```python
from build123d import *

# Parameters (mm, degrees)
SKETCH001_W  = 100
SKETCH001_H  = 80
PAD_DEPTH    = 50
SKETCH_R     = 10
POCKET_DEPTH = 20
SKETCH002_W  = 25
SKETCH002_H  = 50
PAD001_DEPTH = 10


with BuildPart() as part:
    # Sketch001 → Pad (new body)
    with BuildSketch(Plane.XZ):
        Rectangle(SKETCH001_W, SKETCH001_H)
    extrude(amount=-PAD_DEPTH)

    # Sketch → Pocket (cut)
    with BuildSketch(Plane.XZ):
        with Locations((-20, 15)):
            Circle(SKETCH_R)
    extrude(amount=-POCKET_DEPTH, mode=Mode.SUBTRACT)

    # Sketch002 → Pad001 (join)
    with BuildSketch(Plane.XZ):
        with Locations((27.5, -40)):
            Rectangle(SKETCH002_W, SKETCH002_H)
    extrude(amount=-PAD001_DEPTH)


solid = part.part
```
Source: CAD feature listing. Evaluate the final solid. Frame: model axes, mm. A direction names the side the tool comes from. Give positions to 0.01 mm unless a question says otherwise; leave off trailing zeros. Order: outer loops, then holes, each group sorted by start corner. A loop starts at its lowest first (then second) coordinate and runs counter-clockwise, first axis right, second up.
(1) Pull-direction query (X, two-part tool) for faces 1 (the face through (-1, 0, 0)), 2 (the face through (-20, 20, 15)), 3 (the face through (40, 5, -53)); classes: +X half, -X half, draft (parallel to the pull), parting line (faces both ways), or undercut.
(2) Section query A-A (z = 15). Return the cut outline in (x, y), plus the area to 3 significant figures.
(3) Section query C-C (x = -20). Return the cut outline in (y, z), plus the area to 3 significant figures.
(4) Section query B-B (y = 7). Return the cut outline in (x, z).
(5) Material intervals for line 1 along Z through (x, y) = (-20, 13.25); line 2 along Z through (x, y) = (20.5, 43), sorted ascending.
(6) Access query for faces 4 (the face through (-10.46, 9.86, 18)), 5 (the face through (27, 10, -52)), 6 (the face through (-50, 25, -1)), 7 (the face through (15, 5, -53)). Directions: +Z, -Z, +X, -X, +Y, -Y. A direction counts if a zero-diameter tool reaches every point of the face in a straight line with its end or side. Return the directions, or none.
(7) Contact query for flat-ended pins moving along their axis: P1, Ø5, axis at y = 3, z = -55.5, coming from the +X side; P2, Ø7.5, axis at x = 29, z = -56, coming from the +Y side; P3, Ø3, axis at y = 5, z = -49.5, coming from the -X side. Output: stop coordinate, or through.
(8) Section query D-D (y = 17). Return the cut outline in (x, z), plus the area to 3 significant figures.
Outcome:
1. face 1: draft
1. face 2: undercut
1. face 3: +X half
2. outline: (-50, 0) - (-30, 0) - (-30, 20) - (-10, 20) - (-10, 0) - (50, 0) - (50, 50) - (-50, 50) - close
2. area: 4,600 mm2
3. outline: (0, -40) - (50, -40) - (50, 40) - (0, 40) - (0, 25) - (20, 25) - (20, 5) - (0, 5) - close
3. area: 3,600 mm2
4. outline: (-50, -40) - (15, -40) - (15, -65) - (40, -65) - (40, -40) - (50, -40) - (50, 40) - (-50, 40) - close; hole circle Ø20 at (-20, 15)
5. line 1: z = -40 to 5, 25 to 40
5. line 2: z = -40 to 40
6. face 4: -Y
6. face 5: -Z, +X, -X, +Y
6. face 6: +Z, -Z, -X, +Y, -Y
6. face 7: -Z, -X, +Y, -Y
7. P1: stops at x = 40
7. P2: stops at y = 10
7. P3: stops at x = 15
8. outline: (-50, -40) - (50, -40) - (50, 40) - (-50, 40) - close; hole circle Ø20 at (-20, 15)
8. area: 7,690 mm2
